from build123d import *

# Parameters (mm, degrees)
SKETCH1_W           = 42
SKETCH1_H           = 42
BOSS_EXTRUDE1_DEPTH = 2.54
SKETCH2_W           = 42
SKETCH2_H           = 42
BOSS_EXTRUDE2_DEPTH = 12
SKETCH4_R           = 1.813765306
BOSS_EXTRUDE4_DEPTH = 42
SKETCH9_R           = 4.945
SKETCH9_R_2         = 1.945
BOSS_EXTRUDE5_DEPTH = 7
SKETCH10_R          = 1.945
CUT_EXTRUDE1_DEPTH  = 8
FILLET1_R           = 3
FILLET3_R           = 2


with BuildPart() as part:
    # Sketch1 → Boss-Extrude1 (new body)
    with BuildSketch(Plane(origin=(0, 0, 0), x_dir=(1, 0, 0), z_dir=(0, 1, 0))):
        Rectangle(SKETCH1_W, SKETCH1_H)
    extrude(amount=BOSS_EXTRUDE1_DEPTH)

    # Sketch2 → Boss-Extrude2 (add)
    with BuildSketch(Plane(origin=(0, 2.54, 0), x_dir=(1, 0, 0), z_dir=(0, 1, 0))):
        Rectangle(SKETCH2_W, SKETCH2_H)
        with BuildLine():
            Line((-17, 11.522774425), (-17, -11.522774425))
            ThreePointArc((-17, -11.522774425), (-16.869274473, -11.859874356), (-16.545454545, -12.020704023))
            ThreePointArc((-16.545454545, -12.020704023), (-13.464466094, -13.464466094), (-12.020704023, -16.545454545))
            ThreePointArc((-12.020704023, -16.545454545), (-11.859874356, -16.869274473), (-11.522774425, -17))
            Line((-11.522774425, -17), (11.522774425, -17))
            ThreePointArc((11.522774425, -17), (11.859874356, -16.869274473), (12.020704023, -16.545454545))
            ThreePointArc((12.020704023, -16.545454545), (13.464466094, -13.464466094), (16.545454545, -12.020704023))
            ThreePointArc((16.545454545, -12.020704023), (16.869274473, -11.859874356), (17, -11.522774425))
            Line((17, -11.522774425), (17, 11.522774425))
            ThreePointArc((17, 11.522774425), (16.869274473, 11.859874356), (16.545454545, 12.020704023))
            ThreePointArc((16.545454545, 12.020704023), (13.464466094, 13.464466094), (12.020704023, 16.545454545))
            ThreePointArc((12.020704023, 16.545454545), (11.859874356, 16.869274473), (11.522774425, 17))
            Line((11.522774425, 17), (-11.522774425, 17))
            ThreePointArc((-11.522774425, 17), (-11.859874356, 16.869274473), (-12.020704023, 16.545454545))
            ThreePointArc((-12.020704023, 16.545454545), (-13.464466094, 13.464466094), (-16.545454545, 12.020704023))
            ThreePointArc((-16.545454545, 12.020704023), (-16.869274473, 11.859874356), (-17, 11.522774425))
        make_face(mode=Mode.SUBTRACT)
    extrude(amount=BOSS_EXTRUDE2_DEPTH)

    # Sketch4 → Boss-Extrude4 (add)
    with BuildSketch(Plane.ZY.offset(21)):
        with BuildLine():
            Line((7.748459825, 0), (4.708955343, -8.719310622))
            ThreePointArc((4.708955343, -8.719310622), (0, -12.064660663), (-4.708955343, -8.719310622))
            Line((-4.708955343, -8.719310622), (-7.748459825, 0))
            Line((-7.748459825, 0), (7.748459825, 0))
        make_face()
        with Locations((0, -7.077794281)):
            Circle(SKETCH4_R, mode=Mode.SUBTRACT)
    extrude(amount=-BOSS_EXTRUDE4_DEPTH)

    # Sketch9 → Boss-Extrude5 (add)
    with BuildSketch(Plane(origin=(0, 2.54, 0), x_dir=(1, 0, 0), z_dir=(0, 1, 0))):
        with Locations((8, 0)):
            Circle(SKETCH9_R)
        with Locations((8, 0)):
            Circle(SKETCH9_R_2, mode=Mode.SUBTRACT)
        with Locations((-8, 0)):
            Circle(SKETCH9_R)
        with Locations((-8, 0)):
            Circle(SKETCH9_R_2, mode=Mode.SUBTRACT)
    extrude(amount=BOSS_EXTRUDE5_DEPTH)

    # Sketch10 → Cut-Extrude1 (cut)
    with BuildSketch(Plane(origin=(0, 14.54, 0), x_dir=(1, 0, 0), z_dir=(0, 1, 0))):
        with Locations((-17, 17)):
            Circle(SKETCH10_R)
        with Locations((17, 17)):
            Circle(SKETCH10_R)
        with Locations((-17, -17)):
            Circle(SKETCH10_R)
        with Locations((17, -17)):
            Circle(SKETCH10_R)
    extrude(amount=-CUT_EXTRUDE1_DEPTH, mode=Mode.SUBTRACT)

    # Fillet1
    fillet1_edges = [part.edges().sort_by_distance(p)[0] for p in [
        (21, 7.27, 21),
        (-21, 7.27, 21),
        (-21, 7.27, -21),
        (21, 7.27, -21),
    ]]
    fillet(fillet1_edges, radius=FILLET1_R)

    # Fillet3
    fillet3_edges = [part.edges().sort_by_distance(p)[0] for p in [
        (3.055, 2.54, 0),
        (-12.945, 2.54, 0),
    ]]
    fillet(fillet3_edges, radius=FILLET3_R)


solid = part.part
Work out the finished part from the listing and answer in its coordinate system (mm). A direction names the side the tool comes from. Give positions to 0.01 mm unless a question says otherwise; leave off trailing zeros. Write each loop counter-clockwise with the first axis right and the second up, starting at its lowest first coordinate (ties: lowest second). Pieces come first, ordered by that corner, then holes. Notation, with made-up numbers: (51.25, 55) - (70.25, 55) arc R30 cw to (70.25, 90) - close; hole circle Ø11 at (64, 6). An arc over 180 degrees is marked (long way). One line per item, written item: value. Start each with the question number.
1. For faces 5 (the flat face through (-0.294, -4.421, -6.207)), 6 (the flat face through (-5.9, 9.54, -0.1)), determine the directions among +Z, -Z, +X, -X, +Y, -Y from which every point of the face is accessible in a straight line to the end or side of a thin tool.
2. Given pin 1 (6 mm diameter, centred on x = -11.5, z = 5, fed in from +Y); pin 2 (12 mm diameter, centred on x = -15, y = -6.5, fed in from +Z); pin 3 (6 mm diameter, centred on x = 1, z = 13.5, fed in from -Y), each flat-ended and moving along its own axis, determine where each tip first touches the part or whether it passes through.
3. Consider probe 1 along X at (y, z) = (5.75, 0) (3 decimals); probe 2 along Z at (x, y) = (-8, 7.25) (3 decimals); probe 3 along X at (y, z) = (8.5, 6). Determine where each line is inside the solid, lowest interval first.
4. Find section D-D (x = 8). Write down the section's boundary in (y, z) (3 decimals).
5. Find section B-B (y = 3.75). Write down the section's boundary in (x, z) (3 decimals).
6. Find section A-A (y = 9). State how many separate pieces and enclosed holes the cut face has, then the cut area to 3 significant figures.
7. For a pull along X with two mould halves and no side action, classify faces 1 (the cylindrical face through (20.1, 7.37, 20.14)), 2 (the cylindrical face through (13.43, 8.46, 13.5)), 3 (the cylindrical face through (-20.14, 7.17, -20.1)), 4 (the flat face through (-0.29, -4.3, 6.25)) as +X half, -X half, draft (parallel to the pull), parting line (faces both ways), or undercut.
Geometry results:
1. face 5: -Z, +X, -X, -Y
1. face 6: +Y
2. pin 1: y = 9.54
2. pin 2: z = 7.57
2. pin 3: y = 0
3. probe 1: -21 to -17, -12.945 to -9.945, -6.055 to -3.055, 3.055 to 6.055, 9.945 to 12.945, 17 to 21
3. probe 2: -21 to -17, -4.945 to -1.945, 1.945 to 4.945, 17 to 21
3. probe 3: -21 to -17, 17 to 21
4. outline: (-8.719, -4.709) - (0, -7.748) - (0, -21) - (14.54, -21) - (14.54, -17) - (2.54, -17) - (2.54, -6.945) arc R2 cw to (4.54, -4.945) - (9.54, -4.945) - (9.54, -1.945) - (2.54, -1.945) - (2.54, 1.945) - (9.54, 1.945) - (9.54, 4.945) - (4.54, 4.945) arc R2 cw to (2.54, 6.945) - (2.54, 17) - (14.54, 17) - (14.54, 21) - (0, 21) - (0, 7.748) - (-8.719, 4.709) arc R4.987 ccw to start; hole circle Ø3.628 at (-7.078, 0)
5. outline: (-21, -18) arc R3 ccw to (-18, -21) - (18, -21) arc R3 ccw to (21, -18) - (21, 18) arc R3 ccw to (18, 21) - (-18, 21) arc R3 ccw to (-21, 18) - close; circle Ø10.215 at (-8, 0); circle Ø10.215 at (8, 0); hole (-17, -11.523) arc R0.5 ccw to (-16.545, -12.021) arc R5 cw to (-12.021, -16.545) arc R0.5 ccw to (-11.523, -17) - (11.523, -17) arc R0.5 ccw to (12.021, -16.545) arc R5 cw to (16.545, -12.021) arc R0.5 ccw to (17, -11.523) - (17, 11.523) arc R0.5 ccw to (16.545, 12.021) arc R5 cw to (12.021, 16.545) arc R0.5 ccw to (11.523, 17) - (-11.523, 17) arc R0.5 ccw to (-12.021, 16.545) arc R5 cw to (-16.545, 12.021) arc R0.5 ccw to (-17, 11.523) - close; hole circle Ø3.89 at (-8, 0); hole circle Ø3.89 at (8, 0)
6. separate pieces: 3
6. enclosed holes: 7
6. area: 762 mm2
7. face 1: +X half
7. face 2: undercut
7. face 3: -X half
7. face 4: draft
